```python
from build123d import *

# Parameters (mm, degrees)
CYLINDER049_R     = 1.9
CYLINDER049_DEPTH = 10
CYLINDER050_R     = 1.9
CYLINDER050_DEPTH = 10
CYLINDER048_R     = 1.75
CYLINDER048_DEPTH = 10
BOX007_W          = 10
BOX007_H          = 5
BOX007_DEPTH      = 48


with BuildPart() as cylinder049:
    # Cylinder049 → Cylinder049 (new body)
    with BuildSketch(Plane(origin=(-115, 0, -50), x_dir=(1, 0, 0), z_dir=(0, -1, 0))):
        Circle(CYLINDER049_R)
    extrude(amount=CYLINDER049_DEPTH)


with BuildPart() as cylinder050:
    # Cylinder050 → Cylinder050 (new body)
    with BuildSketch(Plane(origin=(-115, 0, -12), x_dir=(1, 0, 0), z_dir=(0, -1, 0))):
        Circle(CYLINDER050_R)
    extrude(amount=CYLINDER050_DEPTH)


with BuildPart() as sidecuts:
    # Cylinder048 → Cylinder048 (new body)
    with BuildSketch(Plane(origin=(-115, 0, -31), x_dir=(1, 0, 0), z_dir=(0, -1, 0))):
        Circle(CYLINDER048_R)
    extrude(amount=CYLINDER048_DEPTH)

    # Fusion017: union Cylinder049, Cylinder050
    add(cylinder049.part)
    add(cylinder050.part)


with BuildPart() as sidecuts_1:
    # Fusion017 placement: moved
    add(sidecuts.part.moved(Location((0, 9.8, 0))))


with BuildPart() as cornerbase:
    # Box007 → Box007 (new body)
    with BuildSketch(Plane(origin=(-120, 0, -55), x_dir=(1, 0, 0), z_dir=(0, 0, 1))):
        with Locations((5, 2.5)):
            Rectangle(BOX007_W, BOX007_H)
    extrude(amount=BOX007_DEPTH)

    # Cut001: cut sideCuts
    add(sidecuts_1.part, mode=Mode.SUBTRACT)


solid = cornerbase.part
```
Could you check a few things on this model? Use its own coordinates, in mm. Coordinates: 2 decimals unless noted, no trailing zeros. Write each loop counter-clockwise with the first axis right and the second up, starting at its lowest first coordinate (ties: lowest second). Pieces come first, ordered by that corner, then holes. Notation, with made-up numbers: (57, -39) - (92, -39) arc R19 cw to (92, -21) - close; hole circle Ø7 at (58.5, 33.5). An arc over 180 degrees is marked (long way). Use a Markdown table: item, result.
Q1. I'm going to push a flat-ended pin straight in: pin 1 Ø1 at (x, z) = (-113.5, -15.5) entering from -Y. Where does the tip first touch, or does it pass through?
Geometry check:
| item | result |
|---|---|
| pin 1 | stops at y = 0 |
Q2. Thinking about a two-plate mould opening in X: for faces 1 (the flat face through (-110, 2, -31)), 2 (the flat face through (-117, 0, -31)), 3 (the cylindrical face through (-116.508, 2.535, -51.156)), which applies, +X half, -X half, draft (parallel to the pull), parting line (faces both ways), or undercut?
Geometry check:
| item | result |
|---|---|
| face 1 | +X half |
| face 2 | draft |
| face 3 | undercut |
Q3. Imagine slicing it at D-D (z = -50). List the corners of the cut face in (x, y) for me, and give its area (3 significant figures).
Geometry check:
| item | result |
|---|---|
| outline | (-120, 0) - (-116.9, 0) - (-116.9, 5) - (-120, 5) - close; (-113.1, 0) - (-110, 0) - (-110, 5) - (-113.1, 5) - close |
| area | 31.0 mm2 |
Q4. Imagine slicing it at C-C (x = -115). List the corners of the cut face in (y, z) for me, and give its area (4 significant figures).
Geometry check:
| item | result |
|---|---|
| outline | (0, -55) - (5, -55) - (5, -51.9) - (0, -51.9) - close; (0, -48.1) - (5, -48.1) - (5, -32.75) - (0, -32.75) - close; (0, -29.25) - (5, -29.25) - (5, -13.9) - (0, -13.9) - close; (0, -10.1) - (5, -10.1) - (5, -7) - (0, -7) - close |
| area | 184.5 mm2 |
Q5. Please list where these lines run through material, in increasing order: L1, parallel to Z at x = -115, y = 1.35; L2, parallel to X at y = 1.25, z = -12; L3, parallel to X at y = 1.45, z = -31.
Geometry check:
| item | result |
|---|---|
| L1 | z = -55 to -51.9, -48.1 to -32.75, -29.25 to -13.9, -10.1 to -7 |
| L2 | x = -120 to -116.9, -113.1 to -110 |
| L3 | x = -120 to -116.75, -113.25 to -110 |
Q6. Imagine slicing it at B-B (y = 2.2). List the corners of the cut face in (x, z) for me, and give its area (3 significant figures).
Geometry check:
| item | result |
|---|---|
| outline | (-120, -55) - (-110, -55) - (-110, -7) - (-120, -7) - close; hole circle Ø3.8 at (-115, -50); hole circle Ø3.8 at (-115, -12); hole circle Ø3.5 at (-115, -31) |
| area | 448 mm2 |
Q7. Imagine slicing it at A-A (z = -31). List the corners of the cut face in (x, y) for me.
Geometry check:
| item | result |
|---|---|
| outline | (-120, 0) - (-116.75, 0) - (-116.75, 5) - (-120, 5) - close; (-113.25, 0) - (-110, 0) - (-110, 5) - (-113.25, 5) - close |
